Source: CAD feature listing. Evaluate the final solid. Frame: model axes, mm. A direction names the side the tool comes from. Round coordinates to 2 decimals unless told otherwise and drop trailing zeros. Loops run counter-clockwise (first coordinate to the right, second up) from the corner with the lowest first, then second, coordinate; pieces in that order, holes last.
(1) Section B-B, the plane y = -2. Return the cut outline in (x, z), plus the area to 3 significant figures.
(2) Section A-A, the plane y = 25. Return the cut outline in (x, z), plus the area to 3 significant figures.
(3) Material intervals for probe 1 along Y at (x, z) = (-84, 2.75); probe 2 along X at (y, z) = (82, 2.2); probe 3 along X at (y, z) = (114, 0.3), sorted ascending.
(4) First-contact query: pin 1 Ø4 at (x, y) = (7.03, 135.05) entering from +Z; pin 2 Ø1.5 at (y, z) = (98.5, 2.5) entering from -X; pin 3 Ø1 at (y, z) = (119.5, 1.5) entering from -X; pin 4 Ø1.5 at (y, z) = (6.5, 0.5) entering from -X. Flat tips, straight axial feed; report the tip coordinate or a pass-through.
(5) Set-up query: faces 1 (the flat face through (61.99, 94.72, 1.97)), 2 (the cylindrical face through (46.618, -26.744, 1.972)). Return all of +Z, -Z, +X, -X, +Y, -Y with unobstructed straight access to the full face (end or side cutting, diameter ignored); none if empty.
(6) Mould query, pull axis Y, two halves, no side actions, for faces 3 (the flat face through (80.03, -11.07, 1.97)), 4 (the flat face through (-74, 81.4, 2)), 5 (the cylindrical face through (-124.062, 135.033, 1.972)). Classes: pulls with the +Y half, pulls with the -Y half, needs draft (parallel to the pull), parting line crosses it, or undercut.
(7) Section C-C, the plane z = 1.75. Count the separate pieces of the cut face and the enclosed holes in it, plus the area to 3 significant figures.
(8) Section D-D, the plane y = 49. Return the cut outline in (x, z).
```python
from build123d import *

# Parameters (mm, degrees)
SKETCH_1_R      = 1.5
SKETCH_1_R_2    = 22.5
SKETCH_1_R_3    = 2.1
SKETCH_1_R_4    = 2
SKETCH_1_W      = 8.4
SKETCH_1_H      = 4.4
SKETCH_1_W_2    = 8.2
SKETCH_1_H_2    = 4.2
EXTRUDE_1_DEPTH = 4


with BuildPart() as part:
    # 草图1 → 凸台-拉伸1 (new body)
    with BuildSketch(Plane.XY):
        with BuildLine():
            Line((7.027428163, -5.002489357), (20.810808237, -16.960441938))
            ThreePointArc((20.810808237, -16.960441938), (47.017847244, -26.746287876), (73.227648339, -16.967842153))
            Line((73.227648339, -16.967842153), (87.027428163, -5.002489357))
            Line((87.027428163, -5.002489357), (87.027428163, 75.054738201))
            Line((87.027428163, 75.054738201), (21.027428163, 141.054738201))
            Line((21.027428163, 141.054738201), (-114.887663771, 141.054738201))
            ThreePointArc((-114.887663771, 141.054738201), (-124.126459096, 134.881572525), (-121.958731583, 123.983670389))
            Line((-121.958731583, 123.983670389), (-90.203942848, 92.228881654))
            Line((-90.203942848, 92.228881654), (7.027428163, -5.002489357))
        make_face()
        with Locations((-52.972571837, 135.054738201)):
            Circle(SKETCH_1_R, mode=Mode.SUBTRACT)
        with Locations((47.027428163, 15.054738201)):
            Circle(SKETCH_1_R_2, mode=Mode.SUBTRACT)
        with Locations(Location((-22.972571837, 135.054738201, 0), (0, 0, 180))):
            Circle(SKETCH_1_R, mode=Mode.SUBTRACT)
        with Locations((7.027428163, 135.054738201)):
            Circle(SKETCH_1_R, mode=Mode.SUBTRACT)
        with Locations(Location((-112.972571837, 135.054738201, 0), (0, 0, 180))):
            Circle(SKETCH_1_R, mode=Mode.SUBTRACT)
        with Locations((-82.972571837, 135.054738201)):
            Circle(SKETCH_1_R, mode=Mode.SUBTRACT)
        with Locations((49.784787476, 103.812097514)):
            Circle(SKETCH_1_R, mode=Mode.SUBTRACT)
        with Locations(Location((70.997990912, 82.598894078, 0), (0, 0, 180))):
            Circle(SKETCH_1_R, mode=Mode.SUBTRACT)
        with Locations(Location((28.571584041, 125.025300949, 0), (0, 0, 180))):
            Circle(SKETCH_1_R, mode=Mode.SUBTRACT)
        with Locations((70.597428163, 38.624738201)):
            Circle(SKETCH_1_R_3, mode=Mode.SUBTRACT)
        with Locations((70.597428163, -8.515261799)):
            Circle(SKETCH_1_R_3, mode=Mode.SUBTRACT)
        with Locations((23.457428163, -8.515261799)):
            Circle(SKETCH_1_R_3, mode=Mode.SUBTRACT)
        with Locations((23.457428163, 38.624738201)):
            Circle(SKETCH_1_R_3, mode=Mode.SUBTRACT)
        with Locations((-83.04451802, 93.554738201)):
            Circle(SKETCH_1_R, mode=Mode.SUBTRACT)
        with Locations((-61.831314585, 72.341534765)):
            Circle(SKETCH_1_R, mode=Mode.SUBTRACT)
        with Locations(Location((-104.257721456, 114.767941637, 0), (0, 0, 180))):
            Circle(SKETCH_1_R, mode=Mode.SUBTRACT)
        with Locations((20.275835807, 57.054738201)):
            Circle(SKETCH_1_R, mode=Mode.SUBTRACT)
        with Locations((-6.58531727, 99.226748532)):
            Circle(SKETCH_1_R_4, mode=Mode.SUBTRACT)
        with Locations((-37.972571837, 135.054738201)):
            Rectangle(SKETCH_1_W, SKETCH_1_H, mode=Mode.SUBTRACT)
        with Locations((-7.972571837, 135.054738201)):
            Rectangle(SKETCH_1_W, SKETCH_1_H, mode=Mode.SUBTRACT)
        with Locations((-97.972571837, 135.054738201)):
            Rectangle(SKETCH_1_W, SKETCH_1_H, mode=Mode.SUBTRACT)
        with Locations((-67.972571837, 135.054738201)):
            Rectangle(SKETCH_1_W, SKETCH_1_H, mode=Mode.SUBTRACT)
        Polygon((55.865905794, 94.619709358), (61.805602756, 88.680012396), (64.916872594, 91.791282234), (58.977175632, 97.730979196), align=None, mode=Mode.SUBTRACT)
        Polygon((34.652702359, 115.832912794), (37.763972196, 118.944182631), (43.703669158, 113.004485669), (40.592399321, 109.893215832), align=None, mode=Mode.SUBTRACT)
        Polygon((-73.852129865, 87.473619883), (-76.963399702, 84.362350046), (-71.02370274, 78.422653084), (-67.912432903, 81.533922921), align=None, mode=Mode.SUBTRACT)
        Polygon((-89.125636339, 102.747126356), (-92.236906176, 99.635856519), (-98.176603138, 105.575553481), (-95.065333301, 108.686823318), align=None, mode=Mode.SUBTRACT)
        with Locations((5.275835807, 57.054738201)):
            Rectangle(SKETCH_1_W_2, SKETCH_1_H_2, mode=Mode.SUBTRACT)
        with Locations((35.275835807, 57.054738201)):
            Rectangle(SKETCH_1_W_2, SKETCH_1_H_2, mode=Mode.SUBTRACT)
    extrude(amount=EXTRUDE_1_DEPTH)


solid = part.part
```
Output values:
1. outline: (4.02, 0) - (32.35, 0) - (32.35, 4) - (4.02, 4) - close; (61.7, 0) - (87.03, 0) - (87.03, 4) - (61.7, 4) - close
1. area: 215 mm2
2. outline: (-22.98, 0) - (26.84, 0) - (26.84, 4) - (-22.98, 4) - close; (67.21, 0) - (87.03, 0) - (87.03, 4) - (67.21, 4) - close
2. area: 279 mm2
3. probe 1: y = 86.02 to 92.4, 94.71 to 133.96, 136.15 to 141.05
3. probe 2: x = -79.98 to -74.6, -68.38 to 69.62, 72.37 to 80.08
3. probe 3: x = -111.98 to -105.55, -102.97 to 36.49, 42.71 to 48.08
4. pin 1: stops at z = 4
4. pin 2: stops at x = -97.23
4. pin 3: stops at x = -117.98
4. pin 4: stops at x = -5.23
5. face 1: +Z, -Z
5. face 2: +Z, -Z, -Y
6. face 3: pulls with the -Y half
6. face 4: undercut
6. face 5: parting line crosses it
7. separate pieces: 1
7. enclosed holes: 28
7. area: 19,100 mm2
8. outline: (-46.98, 0) - (87.03, 0) - (87.03, 4) - (-46.98, 4) - close
